```python
from build123d import *

# Parameters (mm, degrees)
F0_R          = 20
F1_DEPTH      = 9
F2_DEPTH      = 1
F3_DEPTH      = 7
F3_DEPTH_BACK = 1
F4_T4_ANGLE   = 359.64
F4_S5_R       = 19
F4_T6_DEPTH   = 3
F4_T10_ANGLE  = 359.64
F4_S11_R      = 19
F4_T12_DEPTH  = 3
F4_T16_ANGLE  = 359.64
F4_S17_R      = 19
F4_T18_DEPTH  = 3
F4_T22_ANGLE  = 359.64
F4_S23_R      = 19
F4_T24_DEPTH  = 3
F4_T28_ANGLE  = 359.64
F4_S29_R      = 19
F4_T30_DEPTH  = 3
F4_T34_ANGLE  = 359.64
F4_S35_R      = 19
F4_T36_DEPTH  = 3


# Not quite as in the source:
# - a fillet or chamfer that OpenCascade refuses, or shapes differently, is made with other operations: its cross-section is extruded or revolved along the edge and cut away or added


with BuildPart() as f1:
    # F0 (on Top) → F1 (new body)
    with BuildSketch(Plane.XY):
        Circle(F0_R)
        with BuildLine():
            ThreePointArc((16.9315193695, 8.6211166237), (18.4756443463, 4.432895892), (19, 0))
            ThreePointArc((19, 0), (18.4756443463, -4.432895892), (16.9315193695, -8.6211166237))
            ThreePointArc((16.9315193695, -8.6211166237), (16.4544826719, -9.5), (15.9318656899, -10.3525675868))
            ThreePointArc((15.9318656899, -10.3525675868), (9.5, -16.4544826719), (0.9996536796, -18.9736842105))
            ThreePointArc((0.9996536796, -18.9736842105), (0, -19), (-0.9996536796, -18.9736842105))
            ThreePointArc((-0.9996536796, -18.9736842105), (-9.5, -16.4544826719), (-15.9318656899, -10.3525675868))
            ThreePointArc((-15.9318656899, -10.3525675868), (-16.4544826719, -9.5), (-16.9315193695, -8.6211166237))
            ThreePointArc((-16.9315193695, -8.6211166237), (-19, 0), (-16.9315193695, 8.6211166237))
            ThreePointArc((-16.9315193695, 8.6211166237), (-16.4544826719, 9.5), (-15.9318656899, 10.3525675868))
            ThreePointArc((-15.9318656899, 10.3525675868), (-9.5, 16.4544826719), (-0.9996536796, 18.9736842105))
            ThreePointArc((-0.9996536796, 18.9736842105), (0, 19), (0.9996536796, 18.9736842105))
            ThreePointArc((0.9996536796, 18.9736842105), (9.5, 16.4544826719), (15.9318656899, 10.3525675868))
            ThreePointArc((15.9318656899, 10.3525675868), (16.4544826719, 9.5), (16.9315193695, 8.6211166237))
        make_face(mode=Mode.SUBTRACT)
    extrude(amount=F1_DEPTH)

    # F0 (on Top) → F2 (join)
    with BuildSketch(Plane.XY):
        Circle(F0_R)
        with BuildLine():
            ThreePointArc((16.9315193695, 8.6211166237), (18.4756443463, 4.432895892), (19, 0))
            ThreePointArc((19, 0), (18.4756443463, -4.432895892), (16.9315193695, -8.6211166237))
            ThreePointArc((16.9315193695, -8.6211166237), (16.4544826719, -9.5), (15.9318656899, -10.3525675868))
            ThreePointArc((15.9318656899, -10.3525675868), (9.5, -16.4544826719), (0.9996536796, -18.9736842105))
            ThreePointArc((0.9996536796, -18.9736842105), (0, -19), (-0.9996536796, -18.9736842105))
            ThreePointArc((-0.9996536796, -18.9736842105), (-9.5, -16.4544826719), (-15.9318656899, -10.3525675868))
            ThreePointArc((-15.9318656899, -10.3525675868), (-16.4544826719, -9.5), (-16.9315193695, -8.6211166237))
            ThreePointArc((-16.9315193695, -8.6211166237), (-19, 0), (-16.9315193695, 8.6211166237))
            ThreePointArc((-16.9315193695, 8.6211166237), (-16.4544826719, 9.5), (-15.9318656899, 10.3525675868))
            ThreePointArc((-15.9318656899, 10.3525675868), (-9.5, 16.4544826719), (-0.9996536796, 18.9736842105))
            ThreePointArc((-0.9996536796, 18.9736842105), (0, 19), (0.9996536796, 18.9736842105))
            ThreePointArc((0.9996536796, 18.9736842105), (9.5, 16.4544826719), (15.9318656899, 10.3525675868))
            ThreePointArc((15.9318656899, 10.3525675868), (16.4544826719, 9.5), (16.9315193695, 8.6211166237))
        make_face(mode=Mode.SUBTRACT)
        with BuildLine():
            ThreePointArc((16.9315193695, -8.6211166237), (18.4756443463, -4.432895892), (19, 0))
            ThreePointArc((19, 0), (18.4756443463, 4.432895892), (16.9315193695, 8.6211166237))
            ThreePointArc((16.9315193695, 8.6211166237), (15.5884572681, 9), (15.9318656899, 10.3525675868))
            ThreePointArc((15.9318656899, 10.3525675868), (9.5, 16.4544826719), (0.9996536796, 18.9736842105))
            ThreePointArc((0.9996536796, 18.9736842105), (0, 18), (-0.9996536796, 18.9736842105))
            ThreePointArc((-0.9996536796, 18.9736842105), (-9.5, 16.4544826719), (-15.9318656899, 10.3525675868))
            ThreePointArc((-15.9318656899, 10.3525675868), (-15.5884572681, 9), (-16.9315193695, 8.6211166237))
            ThreePointArc((-16.9315193695, 8.6211166237), (-19, 0), (-16.9315193695, -8.6211166237))
            ThreePointArc((-16.9315193695, -8.6211166237), (-15.5884572681, -9), (-15.9318656899, -10.3525675868))
            ThreePointArc((-15.9318656899, -10.3525675868), (-9.5, -16.4544826719), (-0.9996536796, -18.9736842105))
            ThreePointArc((-0.9996536796, -18.9736842105), (0, -18), (0.9996536796, -18.9736842105))
            ThreePointArc((0.9996536796, -18.9736842105), (9.5, -16.4544826719), (15.9318656899, -10.3525675868))
            ThreePointArc((15.9318656899, -10.3525675868), (15.5884572681, -9), (16.9315193695, -8.6211166237))
        make_face()
    extrude(amount=-F2_DEPTH)

    # F0 (on Top) → F3 (join, two sides)
    with BuildSketch(Plane.XY) as f3_sk:
        with BuildLine():
            ThreePointArc((-16.9315193695, 8.6211166237), (-15.5884572681, 9), (-15.9318656899, 10.3525675868))
            ThreePointArc((-15.9318656899, 10.3525675868), (-16.4544826719, 9.5), (-16.9315193695, 8.6211166237))
        make_face()
        with BuildLine():
            ThreePointArc((-0.9996536796, 18.9736842105), (0, 18), (0.9996536796, 18.9736842105))
            ThreePointArc((0.9996536796, 18.9736842105), (0, 19), (-0.9996536796, 18.9736842105))
        make_face()
        with BuildLine():
            ThreePointArc((15.9318656899, 10.3525675868), (15.5884572681, 9), (16.9315193695, 8.6211166237))
            ThreePointArc((16.9315193695, 8.6211166237), (16.4544826719, 9.5), (15.9318656899, 10.3525675868))
        make_face()
        with BuildLine():
            ThreePointArc((15.9318656899, -10.3525675868), (16.4544826719, -9.5), (16.9315193695, -8.6211166237))
            ThreePointArc((16.9315193695, -8.6211166237), (15.5884572681, -9), (15.9318656899, -10.3525675868))
        make_face()
        with BuildLine():
            ThreePointArc((-0.9996536796, -18.9736842105), (0, -19), (0.9996536796, -18.9736842105))
            ThreePointArc((0.9996536796, -18.9736842105), (0, -18), (-0.9996536796, -18.9736842105))
        make_face()
        with BuildLine():
            ThreePointArc((-16.9315193695, -8.6211166237), (-16.4544826719, -9.5), (-15.9318656899, -10.3525675868))
            ThreePointArc((-15.9318656899, -10.3525675868), (-15.5884572681, -9), (-16.9315193695, -8.6211166237))
        make_face()
    extrude(amount=F3_DEPTH)
    extrude(f3_sk.sketch, amount=-F3_DEPTH_BACK)

    # F4: fillet of radius 1 on 6 edges, made by hand


with BuildPart() as f4_tool2:
    # F4_s3 → F4_t4 (revolve)
    with BuildSketch(Plane(origin=(0.0300073325, -0.0515991808, 0), x_dir=(0, 0, 1), z_dir=(0.5027182272, -0.8644503364, 0))):
        with BuildLine():
            ThreePointArc((6, -19.9999062388), (6.7071067812, -19.70701302), (7, -18.9999062388))
            Line((7, -18.9999062388), (7, -19.9999062388))
            Line((7, -19.9999062388), (6, -19.9999062388))
        make_face()
    revolve(axis=Axis((16.4544826719, 9.5, 7), (0, 0, 1)), revolution_arc=F4_T4_ANGLE)

    # F4_s5 → F4_t6 (intersect, symmetric)
    with BuildSketch(Plane.XY.offset(6.5)):
        Circle(F4_S5_R)
    extrude(amount=F4_T6_DEPTH, both=True, mode=Mode.INTERSECT)


with BuildPart() as f1_1:
    add(f1.part)

    # F4_t1: cut F4_tool2
    add(f4_tool2.part, mode=Mode.SUBTRACT)


with BuildPart() as f4_tool8:
    # F4_s9 → F4_t10 (revolve)
    with BuildSketch(Plane(origin=(-0.0296825351, -0.0517867027, 0), x_dir=(0, 0, 1), z_dir=(-0.497276838, -0.8675919239, 0))):
        with BuildLine():
            ThreePointArc((6, -19.9999062388), (6.7071067812, -19.70701302), (7, -18.9999062388))
            Line((7, -18.9999062388), (7, -19.9999062388))
            Line((7, -19.9999062388), (6, -19.9999062388))
        make_face()
    revolve(axis=Axis((16.4544826719, -9.5, 7), (0, 0, 1)), revolution_arc=F4_T10_ANGLE)

    # F4_s11 → F4_t12 (intersect, symmetric)
    with BuildSketch(Plane.XY.offset(6.5)):
        Circle(F4_S11_R)
    extrude(amount=F4_T12_DEPTH, both=True, mode=Mode.INTERSECT)


with BuildPart() as f1_2:
    add(f1_1.part)

    # F4_t7: cut F4_tool8
    add(f4_tool8.part, mode=Mode.SUBTRACT)


with BuildPart() as f4_tool14:
    # F4_s15 → F4_t16 (revolve)
    with BuildSketch(Plane(origin=(-0.0596898677, -0.0001875219, 0), x_dir=(0, 0, 1), z_dir=(-0.9999950652, -0.0031415875, 0))):
        with BuildLine():
            ThreePointArc((6, -19.9999062388), (6.7071067812, -19.70701302), (7, -18.9999062388))
            Line((7, -18.9999062388), (7, -19.9999062388))
            Line((7, -19.9999062388), (6, -19.9999062388))
        make_face()
    revolve(axis=Axis((0, -19, 7), (0, 0, 1)), revolution_arc=F4_T16_ANGLE)

    # F4_s17 → F4_t18 (intersect, symmetric)
    with BuildSketch(Plane.XY.offset(6.5)):
        Circle(F4_S17_R)
    extrude(amount=F4_T18_DEPTH, both=True, mode=Mode.INTERSECT)


with BuildPart() as f1_3:
    add(f1_2.part)

    # F4_t13: cut F4_tool14
    add(f4_tool14.part, mode=Mode.SUBTRACT)


with BuildPart() as f4_tool20:
    # F4_s21 → F4_t22 (revolve)
    with BuildSketch(Plane(origin=(-0.0300073325, 0.0515991808, 0), x_dir=(0, 0, 1), z_dir=(-0.5027182272, 0.8644503364, 0))):
        with BuildLine():
            ThreePointArc((6, -19.9999062388), (6.7071067812, -19.70701302), (7, -18.9999062388))
            Line((7, -18.9999062388), (7, -19.9999062388))
            Line((7, -19.9999062388), (6, -19.9999062388))
        make_face()
    revolve(axis=Axis((-16.4544826719, -9.5, 7), (0, 0, 1)), revolution_arc=F4_T22_ANGLE)

    # F4_s23 → F4_t24 (intersect, symmetric)
    with BuildSketch(Plane.XY.offset(6.5)):
        Circle(F4_S23_R)
    extrude(amount=F4_T24_DEPTH, both=True, mode=Mode.INTERSECT)


with BuildPart() as f1_4:
    add(f1_3.part)

    # F4_t19: cut F4_tool20
    add(f4_tool20.part, mode=Mode.SUBTRACT)


with BuildPart() as f4_tool26:
    # F4_s27 → F4_t28 (revolve)
    with BuildSketch(Plane(origin=(0.0296825351, 0.0517867027, 0), x_dir=(0, 0, 1), z_dir=(0.497276838, 0.8675919239, 0))):
        with BuildLine():
            ThreePointArc((6, -19.9999062388), (6.7071067812, -19.70701302), (7, -18.9999062388))
            Line((7, -18.9999062388), (7, -19.9999062388))
            Line((7, -19.9999062388), (6, -19.9999062388))
        make_face()
    revolve(axis=Axis((-16.4544826719, 9.5, 7), (0, 0, 1)), revolution_arc=F4_T28_ANGLE)

    # F4_s29 → F4_t30 (intersect, symmetric)
    with BuildSketch(Plane.XY.offset(6.5)):
        Circle(F4_S29_R)
    extrude(amount=F4_T30_DEPTH, both=True, mode=Mode.INTERSECT)


with BuildPart() as f1_5:
    add(f1_4.part)

    # F4_t25: cut F4_tool26
    add(f4_tool26.part, mode=Mode.SUBTRACT)


with BuildPart() as f4_tool32:
    # F4_s33 → F4_t34 (revolve)
    with BuildSketch(Plane(origin=(0.0596898677, 0.0001875219, 0), x_dir=(0, 0, 1), z_dir=(0.9999950652, 0.0031415875, 0))):
        with BuildLine():
            ThreePointArc((6, -19.9999062388), (6.7071067812, -19.70701302), (7, -18.9999062388))
            Line((7, -18.9999062388), (7, -19.9999062388))
            Line((7, -19.9999062388), (6, -19.9999062388))
        make_face()
    revolve(axis=Axis((0, 19, 7), (0, 0, 1)), revolution_arc=F4_T34_ANGLE)

    # F4_s35 → F4_t36 (intersect, symmetric)
    with BuildSketch(Plane.XY.offset(6.5)):
        Circle(F4_S35_R)
    extrude(amount=F4_T36_DEPTH, both=True, mode=Mode.INTERSECT)


with BuildPart() as f1_6:
    add(f1_5.part)

    # F4_t31: cut F4_tool32
    add(f4_tool32.part, mode=Mode.SUBTRACT)


solid = f1_6.part
```
Can you work these out from the model? Positions are in its coordinate system, mm. A direction names the side the tool comes from. Coordinates: 2 decimals unless noted, no trailing zeros. Loops run counter-clockwise (first coordinate to the right, second up) from the corner with the lowest first, then second, coordinate; pieces in that order, holes last. Notation, with made-up numbers: (-14, 65.25) - (13, 65.25) arc R7 ccw to (13, 76.25) - close; hole circle Ø5 at (48.25, 2.25). An arc over 180 degrees is marked (long way). Use a Markdown table: item, result.
Item 1: I want a section at B-B on y = 3. Please give me the cut outline in (x, z), and give its area (3 significant figures).
Numbers:
| item | result |
|---|---|
| outline | (-19.77, -1) - (19.77, -1) - (19.77, 9) - (18.76, 9) - (18.76, 0) - (-18.76, 0) - (-18.76, 9) - (-19.77, 9) - close |
| area | 57.8 mm2 |
Item 2: I want a section at C-C on x = 7. Please give me the cut outline in (y, z) (3 decimals), and give its area (3 significant figures).
Numbers:
| item | result |
|---|---|
| outline | (-18.735, -1) - (18.735, -1) - (18.735, 9) - (17.664, 9) - (17.664, 0) - (-17.664, 0) - (-17.664, 9) - (-18.735, 9) - close |
| area | 56.8 mm2 |
Item 3: I want a section at A-A on z = 3. Please give me the cut outline in (x, y), and give its area (3 significant figures).
Numbers:
| item | result |
|---|---|
| outline | circle Ø40 at (0, 0); hole (-16.93, -8.62) arc R1 cw to (-15.93, -10.35) arc R19 ccw to (-1, -18.97) arc R1 cw to (1, -18.97) arc R19 ccw to (15.93, -10.35) arc R1 cw to (16.93, -8.62) arc R19 ccw to (16.93, 8.62) arc R1 cw to (15.93, 10.35) arc R19 ccw to (1, 18.97) arc R1 cw to (-1, 18.97) arc R19 ccw to (-15.93, 10.35) arc R1 cw to (-16.93, 8.62) arc R19 ccw to start |
| area | 132 mm2 |
Item 4: Will these pins go through, and if not, where does the flat tip stop? pin 1 (2 mm diameter, centred on y = -6.5, z = 3.5, fed in from +X); pin 2 (2 mm diameter, centred on x = -7, z = 4, fed in from -Y); pin 3 (3 mm diameter, centred on y = 15, z = 3, fed in from +X).
Numbers:
| item | result |
|---|---|
| pin 1 | stops at x = 19.23 |
| pin 2 | stops at y = -19.08 |
| pin 3 | stops at x = 14.76 |
Item 5: If I drill on probe 1 along Z at (x, y) = (5, -9); probe 2 along X at (y, z) = (12, 8.5); probe 3 along Y at (x, z) = (8.5, 4.75), over which ranges is the centre line in solid material (lowest first)? Write a range as from..to.
Numbers:
| item | result |
|---|---|
| probe 1 | z = -1..0 |
| probe 2 | x = -16..-14.73, 14.73..16 |
| probe 3 | y = -18.1..-16.99, 16.99..18.1 |
Item 6: For faces 4 (the face through (0, 0, 0)), 5 (the face through (0, 0, -1)), which set-ups out of +Z, -Z, +X, -X, +Y, -Y let a thin tool reach every point of the face, with its end or its side?
Numbers:
| item | result |
|---|---|
| face 4 | +Z |
| face 5 | -Z, +X, -X, +Y, -Y |
Item 7: We'd pull the mould along X, two halves only. Please class faces 1 (the face through (18, -7, 9)), 2 (the face through (-4.336, -19.524, 4.07)), 3 (the face through (-15.6, 8.98, 2.96)): released by +X, released by -X, zero draft, split by the parting line, or undercut.
Numbers:
| item | result |
|---|---|
| face 1 | zero draft |
| face 2 | split by the parting line |
| face 3 | undercut |
